For this review, take the finished solid that the model builds, in its own axes (mm). Coordinates: 2 decimals unless noted, no trailing zeros. Write each loop counter-clockwise with the first axis right and the second up, starting at its lowest first coordinate (ties: lowest second). Pieces come first, ordered by that corner, then holes. Notation, with made-up numbers: (83, 84.25) -> (94, 84.25) arc R36 cw to (94, 118.25) -> close; hole circle Ø5 at (55.25, 22). An arc over 180 degrees is marked (long way). One line per item, written item: value. Start each with the question number.
1) For probe 1 along X at (y, z) = (150.5, 1.55); probe 2 along Y at (x, z) = (84, 0.2); probe 3 along X at (y, z) = (149.75, 1.5), list the stretches that pass through material, from the lowest coordinate up. Write a range as from..to.
2) Add section C-C (x = 38). State the section outline as (y, z) points.
3) Add section A-A (z = 0.6). State the section outline as (x, y) points, and give its area (3 significant figures).
4) For pin 1 Ø4 at (x, y) = (56, 149) entering from -Z; pin 2 Ø2.5 at (x, y) = (9.78, 150.82) entering from -Z; pin 3 Ø1.5 at (y, z) = (153, 2.5) entering from -X, all flat-tipped, find the tip position at first contact; note any pin that passes through.
5) Add section B-B (x = 13). State the section outline as (y, z) points.
from build123d import *

# Parameters (mm, degrees)
SKETCH_1_R      = 1.5
EXTRUDE_1_DEPTH = 3


with BuildPart() as part:
    # 草圖1 → 填料-伸長1 (new body)
    with BuildSketch(Plane.XY):
        with BuildLine():
            Line((28.43076164, 146.77282614), (84.081040564, 147.012256058))
            ThreePointArc((84.081040564, 147.012256058), (85.747384171, 146.841113393), (87.341537057, 146.326655031))
            ThreePointArc((87.341537057, 146.326655031), (88.27023729, 146.018781), (89.213720756, 145.759726003))
            ThreePointArc((89.213720756, 145.759726003), (95.537127916, 152.779296104), (87.206898507, 157.236550922))
            ThreePointArc((87.206898507, 157.236550922), (85.625904315, 156.682898569), (83.964278534, 156.470593769))
            Line((83.964278534, 156.470593769), (9.689328559, 154.823969204))
            ThreePointArc((9.689328559, 154.823969204), (6.708309072, 153.340450311), (5.825145652, 150.129947568))
            ThreePointArc((5.825145652, 150.129947568), (6.818352081, 148.234093963), (8.49347494, 146.901921561))
            ThreePointArc((8.49347494, 146.901921561), (9.408892458, 146.744827981), (10.336347773, 146.694885369))
            Line((10.336347773, 146.694885369), (28.43076164, 146.77282614))
        make_face()
        with Locations((89.77184724, 151.812467685)):
            Circle(SKETCH_1_R, mode=Mode.SUBTRACT)
        with Locations((9.777984027, 150.8249518)):
            Circle(SKETCH_1_R, mode=Mode.SUBTRACT)
    extrude(amount=EXTRUDE_1_DEPTH)


solid = part.part
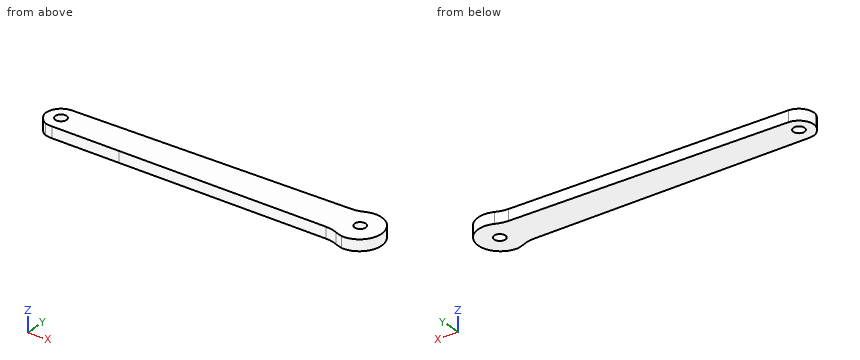
Numbers:
1. probe 1: 5.79..8.31, 11.24..89.05, 90.5..95.5
1. probe 2: 147.01..156.47
1. probe 3: 5.95..8.73, 10.82..95.29
2. outline: (146.81, 0) -> (155.45, 0) -> (155.45, 3) -> (146.81, 3) -> close
3. outline: (5.83, 150.13) arc R5.18 ccw to (8.49, 146.9) arc R8 ccw to (10.34, 146.69) -> (28.43, 146.77) -> (84.08, 147.01) arc R8 cw to (87.34, 146.33) arc R18.77 ccw to (89.21, 145.76) arc R6 ccw (long way) to (87.21, 157.24) arc R8 cw to (83.96, 156.47) -> (9.69, 154.82) arc R4.08 ccw to start; hole circle Ø3 at (9.78, 150.82); hole circle Ø3 at (89.77, 151.81)
3. area: 780 mm²
4. pin 1: z = 0
4. pin 2: through
4. pin 3: x = 6.07
5. outline: (146.71, 0) -> (154.9, 0) -> (154.9, 3) -> (146.71, 3) -> close
